Source: three-view drawing plus pictorial views. Frame: mm from the lowest corner of the part. Round coordinates to 2 decimals unless told otherwise and drop trailing zeros. Write each loop counter-clockwise with the first axis right and the second up, starting at its lowest first coordinate (ties: lowest second). Pieces come first, ordered by that corner, then holes. Notation, with made-up numbers: (11.5, -10.5) -> (37.5, -10.5) arc R27 cw to (37.5, 25.5) -> close; hole circle Ø5 at (-30.5, -37). An arc over 180 degrees is marked (long way). Put each result on its own line as item: value.
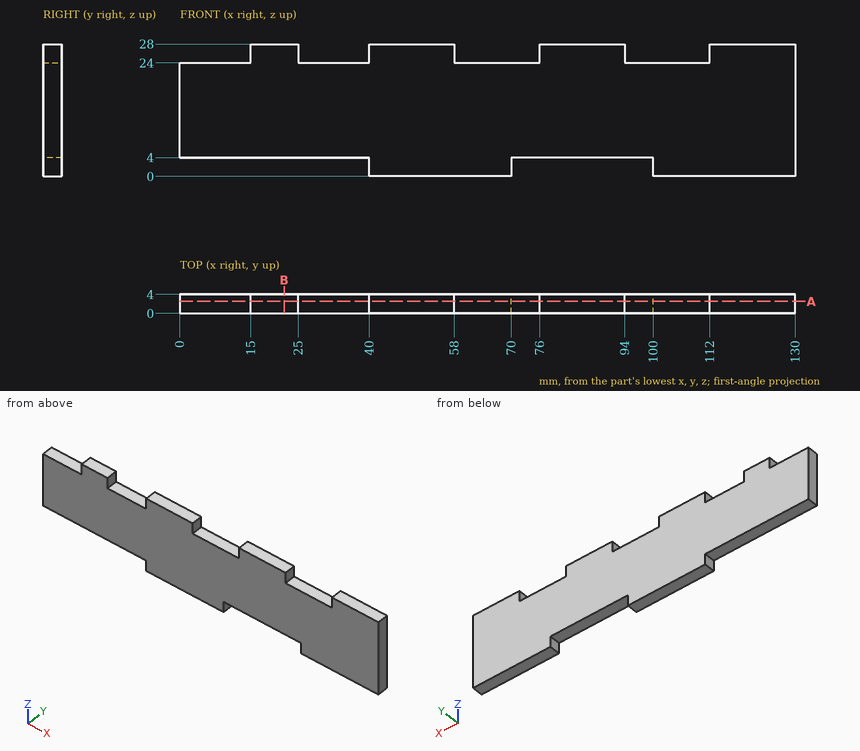
Q1. Pin query (flat end, axial travel): pin 1 (1.2 mm diameter, centred on x = 78.5, y = 2, fed in from -Z); pin 2 (1.2 mm diameter, centred on x = 36, y = 2, fed in from +Z). Return the tip coordinate at first contact, or that it passes through.
Ans:
pin 1: stops at z = 4
pin 2: stops at z = 24
Q2. Material intervals for line 1 (X direction, y = 3.7, z = 2.75); line 2 (Z direction, x = 81.5, y = 3.45); line 3 (Z direction, x = 30, y = 3.65), sorted ascending. Write a range as [from, to].
Ans:
line 1: x = [40, 70], [100, 130]
line 2: z = [4, 28]
line 3: z = [4, 24]
Q3. Cut plane A-A on y = 2.55. Output: boundary loops of the cut face in (x, z), and give its area (3 significant figures).
Ans:
outline: (0, 4) -> (40, 4) -> (40, 0) -> (70, 0) -> (70, 4) -> (100, 4) -> (100, 0) -> (130, 0) -> (130, 28) -> (112, 28) -> (112, 24) -> (94, 24) -> (94, 28) -> (76, 28) -> (76, 24) -> (58, 24) -> (58, 28) -> (40, 28) -> (40, 24) -> (25, 24) -> (25, 28) -> (15, 28) -> (15, 24) -> (0, 24) -> close
area: 3,100 mm^2
Q4. Cut plane B-B on x = 22. Output: boundary loops of the cut face in (y, z).
Ans:
outline: (0, 4) -> (4, 4) -> (4, 28) -> (0, 28) -> close
